Check sheet for the modelled part. Datum: model origin and axes. Units: mm. A direction names the side the tool comes from. Coordinates: 2 decimals unless noted, no trailing zeros. Loops run counter-clockwise (first coordinate to the right, second up) from the corner with the lowest first, then second, coordinate; pieces in that order, holes last. Notation, with made-up numbers: M 10,5.5 L 69,5.5 A19 ccw 69,13.5 Z; hole C -18,86 d6. An arc over 180 degrees is marked long. Answer as CSV lines item,"result". Start each with the question number.
from build123d import *

# Parameters (mm, degrees)
F1_DEPTH      = 10
F1_DEPTH_BACK = 10
F3_D          = 4
F5_D          = 4
F5_DEPTH      = 18.2076214093
F7_D          = 8
F8_R          = 3
F9_R          = 5
F11_D         = 4
F13_DEPTH     = 25


with BuildPart() as f1:
    # F0 (on Front) → F1 (new body, two sides)
    with BuildSketch(Plane.XZ) as f1_sk:
        Polygon((-40.2948366535, -6.0925860852), (-36.1803398875, -11.7557050458), (-20, 0), (15, 0), (26.7557050458, -16.1803398875), (32.4188240065, -12.0658431215), (18.5666781465, 7), (-22.2744378736, 7), align=None)
    extrude(amount=F1_DEPTH)
    extrude(f1_sk.sketch, amount=-F1_DEPTH_BACK)

    # F3 (through all)
    with Locations(Plane(origin=(-6.9098300563, 0, 9.510565163), x_dir=(0.8090169944, 0, 0.5877852523), z_dir=(0.5877852523, 0, -0.8090169944))):
        with Locations((0, -37.8532769899), (0, -24.0082326065), (-30.1803398875, 0), (-21.1803398875, 0)):
            Hole(F3_D / 2)

    # F5 (through all, one way)
    with BuildSketch(Plane(origin=(9.8176274578, 0, 7.1329238722), x_dir=(0, -1, 0), z_dir=(-0.8090169944, 0, -0.5877852523))):
        with Locations((16.0583042515, 0), (-6.1736582538, 0)):
            Circle(F5_D / 2)
    extrude(amount=-F5_DEPTH, mode=Mode.SUBTRACT)

    # F7 (through all)
    with Locations(Plane(origin=(0, 0, 0), x_dir=(1, 0, 0), z_dir=(0, 0, -1))):
        with Locations((0, 0)):
            Hole(F7_D / 2)

    # F8
    f8_edges = [f1.edges().sort_by_distance(p)[0] for p in [
        (-36.18034, 0, -11.755705),
        (26.755705, 0, -16.18034),
    ]]
    fillet(f8_edges, radius=F8_R)

    # F9
    f9_edges = [f1.edges().sort_by_distance(p)[0] for p in [
        (-20, 0, 0),
        (15, 0, 0),
    ]]
    fillet(f9_edges, radius=F9_R)

    # F11 (through all)
    with Locations(Plane(origin=(9.8176274578, 0, 7.1329238722), x_dir=(0, -1, 0), z_dir=(-0.8090169944, 0, -0.5877852523))):
        with Locations((0, -15.1145784184), (0, -22.5539375097)):
            Hole(F11_D / 2)

    # F12 (on face) → F13 (cut)
    with BuildSketch(Plane(origin=(0, 0, 0), x_dir=(1, 0, 0), z_dir=(0, 0, -1))):
        with BuildLine():
            Line((-4, 10), (-4, 0))
            ThreePointArc((-4, 0), (0, 4), (4, 0))
            Line((4, 0), (4, 10))
            Line((4, 10), (-4, 10))
        make_face()
    extrude(amount=-F13_DEPTH, mode=Mode.SUBTRACT)


solid = f1.part
Item 1: Release check for a two-part mould opening along Z. For faces 4 (the face through (14.69, -0.14, -0.53)), 5 (the face through (-31.8, -0.09, -4.18)), 6 (the face through (-6, 0, 7)) record: released by +Z, released by -Z, zero draft, split by the parting line, or undercut.
Item 2: Sectioned sample at B-B, the plane x = 14. Record the boundary of the cut face in (y, z), and give its area (3 significant figures).
Item 3: Material ranges on line 1 (X direction, y = 3.5, z = -6.5) (3 decimals); line 2 (X direction, y = -4.25, z = -2.25); line 3 (Z direction, x = -17, y = -2.25), recorded low to high. Write a range as from..to.
Item 4: Sectioned sample at A-A, the plane x = 0. Record the boundary of the cut face in (y, z).
Item 5: Set-up check for faces 1 (the face through (-7, 0, 0)), 2 (the face through (-4, -5, 3)), 3 (the face through (11.8, 6.2, 6.1)): record each of +Z, -Z, +X, -X, +Y, -Y from which the full face is reachable in a straight line by a thin tool's end or side.
Item 6: Go/stop test with flat-tipped pins: pin 1 (5 mm diameter, centred on y = -5.5, z = -0.5, fed in from +X); pin 2 (8 mm diameter, centred on y = -4.5, z = -2, fed in from -X); pin 3 (1 mm diameter, centred on x = -29, y = -1.5, fed in from +Z). Record where each tip stops, or that it passes through.
Reply:
1,face 4,"released by -Z"
1,face 5,"undercut"
1,face 6,"released by +Z"
2,outline,"M -10,-0.25 L 10,-0.25 L 10,7 L -10,7 Z"
2,area,"145 mm²"
3,line 1,"-39.999..-28.946, 19.723..28.375"
3,line 2,"-35.01..-23.1, 16.63..25.29"
3,line 3,"0..7"
4,outline,"M 4,0 L 10,0 L 10,7 L 4,7 Z"
5,face 1,"-Z, +Y, -Y"
5,face 2,"+Z, -Z, -Y"
5,face 3,"+Z"
6,pin 1,"x = 25.83"
6,pin 2,"x = -40.17"
6,pin 3,"z = 2.34"
